from build123d import *

# Parameters (mm, degrees)
F1_DEPTH = 641.35
F2_R     = 2.54
F4_DEPTH = 1.27


# Not quite as in the source:
# - a pattern or mirror of a feature is missing from the dataset's text; its kind, count and spacing are read off the source's solid


with BuildPart() as f1:
    # F0 (on Right) → F1 (new body, symmetric)
    with BuildSketch(Plane.YZ):
        Polygon((-1.27, 0), (0, 0), (0, 50.8), (1206.5, 50.8), (1206.5, -1155.7), (1207.77, -1155.7), (1207.77, 52.07), (-1.27, 52.07), align=None)
    extrude(amount=F1_DEPTH, both=True)

    # F2
    f2_edges = [f1.edges().sort_by_distance(p)[0] for p in [
        (0, 1207.77, 52.07),
    ]]
    fillet(f2_edges, radius=F2_R)

    # F3 (on face) → F4 (join)
    with BuildSketch(Plane.YZ.offset(641.35)):
        with BuildLine():
            Line((1205.23, 52.07), (-1.27, 52.07))
            Line((-1.27, 52.07), (30.48, 20.32))
            Line((30.48, 20.32), (1172.2684317215, 20.32))
            Line((1172.2684317215, 20.32), (1204.2542837185, 50.8))
            Line((1204.2542837185, 50.8), (1206.5, 50.8))
            Line((1206.5, 50.8), (1206.5, 48.5542837185))
            Line((1206.5, 48.5542837185), (1176.02, 19.5092421769))
            Line((1176.02, 19.5092421769), (1176.02, -1123.95))
            Line((1176.02, -1123.95), (1207.77, -1155.7))
            Line((1207.77, -1155.7), (1207.77, -1123.95))
            Line((1207.77, -1123.95), (1207.77, 49.53))
            ThreePointArc((1207.77, 49.53), (1207.0260512242, 51.3260512242), (1205.23, 52.07))
        make_face()
    f4 = extrude(amount=F4_DEPTH)

    # F4_copies: F4 across plane
    add(f4.mirror(Plane(origin=(0, 0, 0), x_dir=(0, 0, -1), z_dir=(-1, 0, 0))))


solid = f1.part
Could you check a few things on this model? Use its own coordinates, in mm. Give positions to 0.01 mm unless a question says otherwise; leave off trailing zeros. Order: outer loops, then holes, each group sorted by start corner. A loop starts at its lowest first (then second) coordinate and runs counter-clockwise, first axis right, second up. Notation, with made-up numbers: M 79.25,-20.75 L 89.25,-20.75 A30 cw 89.25,18.25 Z; hole C -17,-39 d3. An arc over 180 degrees is marked long. One line per question, with ' | ' between items.
1. I want a section at C-C (y = 524). List the corners of the cut face in (x, z) for me.
Results:
outline: M -642.62,20.32 L -641.35,20.32 L -641.35,50.8 L 641.35,50.8 L 641.35,20.32 L 642.62,20.32 L 642.62,52.07 L -642.62,52.07 Z
2. I'm going to push flat-ended pins straight in: pin 1 (0.6 mm diameter, centred on x = 642.5, z = -307.5, fed in from -Y); pin 2 (10 mm diameter, centred on x = 190, y = 469.5, fed in from -Z); pin 3 (1.4 mm diameter, centred on x = 642, y = 603.5, fed in from -Z). Where does each tip first touch, or does it pass through?
Results:
pin 1: y = 1176.02 | pin 2: z = 50.8 | pin 3: z = 20.32
3. I want a section at A-A (x = 138.5). List the corners of the cut face in (y, z) for me, and give its area (3 significant figures).
Results:
outline: M -1.27,0 L 0,0 L 0,50.8 L 1206.5,50.8 L 1206.5,-1155.7 L 1207.77,-1155.7 L 1207.77,49.53 A2.54 ccw 1205.23,52.07 L -1.27,52.07 Z | area: 3,130 mm²
4. We'd pull the mould along X, two halves only. Please class faces 1 (the face through (-642.62, 869, 33)), 2 (the face through (9, -1.27, 26)), 3 (the face through (9, 595, 50.8)), 4 (the face through (9, 1206.5, -544)): +X half, -X half, draft (parallel to the pull), parting line (faces both ways), or undercut.
Results:
face 1: -X half | face 2: draft | face 3: undercut | face 4: undercut
5. If I drill on line 1 (Y direction, x = -241, z = -362); line 2 (Z direction, x = -529, y = 638), over which ranges is the centre line in solid material (lowest first)?
Results:
line 1: 1206.5 to 1207.77 | line 2: 50.8 to 52.07
6. I want a section at B-B (z = -534.5). List the corners of the cut face in (x, y) for me.
Results:
outline: M -642.62,1176.02 L -641.35,1176.02 L -641.35,1206.5 L 641.35,1206.5 L 641.35,1176.02 L 642.62,1176.02 L 642.62,1207.77 L -642.62,1207.77 Z
